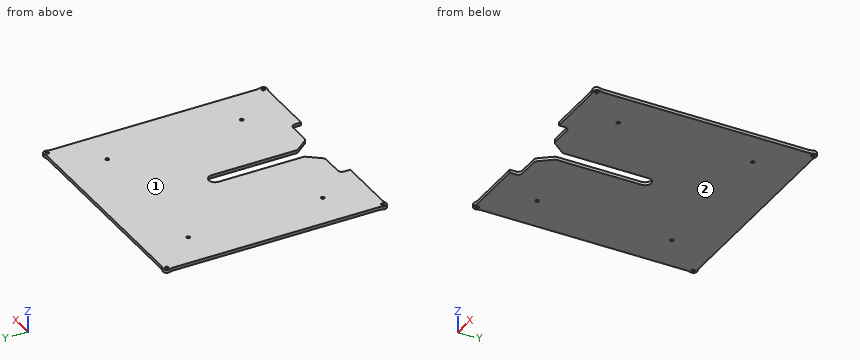
from build123d import *

# Parameters (mm, degrees)
SKETCH1_R           = 1.6
BOSS_EXTRUDE1_DEPTH = 3
CUT_EXTRUDE1_DEPTH  = 4
CUT_EXTRUDE3_DEPTH  = 4
FILLET1_R           = 4
SKETCH3_R           = 1.6
CUT_EXTRUDE2_DEPTH  = 4


with BuildPart() as part:
    # Sketch1 → Boss-Extrude1 (new body)
    with BuildSketch(Plane.XY):
        with BuildLine():
            Line((-107, 98.923010333), (-107, -98.923010333))
            ThreePointArc((-107, -98.923010333), (-107.201661971, -101.11372249), (-107.799869959, -103.230804092))
            ThreePointArc((-107.799869959, -103.230804092), (-107, -107), (-103.230804092, -107.799869959))
            ThreePointArc((-103.230804092, -107.799869959), (-101.11372249, -107.201661971), (-98.923010333, -107))
            Line((-98.923010333, -107), (-43, -107))
            Line((-43, -107), (-43, -101))
            ThreePointArc((-43, -101), (-41.828427125, -98.171572875), (-39, -97))
            Line((-39, -97), (39, -97))
            ThreePointArc((39, -97), (41.828427125, -98.171572875), (43, -101))
            Line((43, -101), (43, -107))
            Line((43, -107), (98.923010333, -107))
            ThreePointArc((98.923010333, -107), (101.11372249, -107.201661971), (103.230804092, -107.799869959))
            ThreePointArc((103.230804092, -107.799869959), (107, -107), (107.799869959, -103.230804092))
            ThreePointArc((107.799869959, -103.230804092), (107.201661971, -101.11372249), (107, -98.923010333))
            Line((107, -98.923010333), (107, 98.923010333))
            ThreePointArc((107, 98.923010333), (107.201661971, 101.11372249), (107.799869959, 103.230804092))
            ThreePointArc((107.799869959, 103.230804092), (107, 107), (103.230804092, 107.799869959))
            ThreePointArc((103.230804092, 107.799869959), (101.11372249, 107.201661971), (98.923010333, 107))
            Line((98.923010333, 107), (-98.923010333, 107))
            ThreePointArc((-98.923010333, 107), (-101.11372249, 107.201661971), (-103.230804092, 107.799869959))
            ThreePointArc((-103.230804092, 107.799869959), (-107, 107), (-107.799869959, 103.230804092))
            ThreePointArc((-107.799869959, 103.230804092), (-107.201661971, 101.11372249), (-107, 98.923010333))
        make_face()
        with Locations((-104.5, -104.5)):
            Circle(SKETCH1_R, mode=Mode.SUBTRACT)
        with Locations((-104.5, 104.5)):
            Circle(SKETCH1_R, mode=Mode.SUBTRACT)
        with Locations((104.5, 104.5)):
            Circle(SKETCH1_R, mode=Mode.SUBTRACT)
        with Locations((104.5, -104.5)):
            Circle(SKETCH1_R, mode=Mode.SUBTRACT)
    extrude(amount=BOSS_EXTRUDE1_DEPTH)

    # Sketch2 → Cut-Extrude1 (cut, through all)
    with BuildSketch(Plane(origin=(0, 0, 0), x_dir=(-1, 0, 0), z_dir=(0, 0, -1))):
        with BuildLine():
            Line((6, -97), (-6, -97))
            Line((-6, -97), (-6, 0))
            ThreePointArc((-6, 0), (0, 6), (6, 0))
            Line((6, 0), (6, -97))
        make_face()
    extrude(amount=-CUT_EXTRUDE1_DEPTH, mode=Mode.SUBTRACT)

    # Sketch4 → Cut-Extrude3 (cut, through all)
    with BuildSketch(Plane.XY.offset(3)):
        Polygon((-17, -97), (17, -97), (6, -83), (-6, -83), align=None)
    extrude(amount=-CUT_EXTRUDE3_DEPTH, mode=Mode.SUBTRACT)

    # Fillet1
    fillet1_edges = [part.edges().sort_by_distance(p)[0] for p in [
        (-17, -97, 1.5),
        (-6, -83, 1.5),
        (6, -83, 1.5),
        (17, -97, 1.5),
    ]]
    fillet(fillet1_edges, radius=FILLET1_R)

    # Sketch3 → Cut-Extrude2 (cut, through all)
    with BuildSketch(Plane.XY.offset(3)):
        with Locations((-71, 65)):
            Circle(SKETCH3_R)
        with Locations((71, 65)):
            Circle(SKETCH3_R)
        with Locations((71, -65)):
            Circle(SKETCH3_R)
        with Locations((-71, -65)):
            Circle(SKETCH3_R)
    extrude(amount=-CUT_EXTRUDE2_DEPTH, mode=Mode.SUBTRACT)


solid = part.part
Verification items for the finished model (mm, model axes). Face numbers are marked on the shaded views. Give positions to 0.01 mm unless a question says otherwise; leave off trailing zeros. Order: outer loops, then holes, each group sorted by start corner. A loop starts at its lowest first (then second) coordinate and runs counter-clockwise, first axis right, second up. Notation, with made-up numbers: M 89,-24 L 136,-24 A9 cw 136,-18 Z; hole C -14.75,73 d11. An arc over 180 degrees is marked long. Answer as a JSON object with one key per item and string values. Group by question number.
1) Cross-section at B-B (z = 0.9). Give the number of separate pieces and of enclosed holes in the cut face, then the cut area to 3 significant figures.
2) Mould release check, pull along Z, two halves, no side actions. Record for the marked faces 1 and 2: released by +Z, released by -Z, zero draft, split by the parting line, or undercut.
3) Cross-section at D-D (y = -93). Enter the section's corners in (x, z), then the cut area to 3 significant figures.
4) Cross-section at C-C (x = 35). Enter the section's corners in (y, z).
5) Scan lines: line 1 along X through (y, z) = (-104.5, 2.3); line 2 along Y through (x, z) = (71, 1.6); line 3 along X through (y, z) = (-65, 1.7). Record each from-to range of solid material in increasing order. Write a range as [from, to].
6) Depth check by flat-ended pin: pin 1 Ø3.5 at (x, y) = (-104.5, 104.5) entering from +Z; pin 2 Ø3 at (x, y) = (-71, -65) entering from +Z; pin 3 Ø0.9 at (y, z) = (-102.5, 2) entering from -X; pin 4 Ø0.9 at (x, z) = (-33.5, 1.5) entering from -Y. Enter the tip coordinate at first touch or a pass-through.
7) Cross-section at A-A (y = -27.5). Enter the section's corners in (x, z), then the cut area to 3 significant figures.
Result sheet:
{
 "1": {"separate pieces": "1", "enclosed holes": "8", "area": "43,500 mm2"},
 "2": {"face 1": "released by +Z", "face 2": "released by -Z"},
 "3": {"outline": "M -107,0 L -13.86,0 L -13.86,3 L -107,3 Z; M 13.86,0 L 107,0 L 107,3 L 13.86,3 Z", "area": "559 mm2"},
 "4": {"outline": "M -97,0 L 107,0 L 107,3 L -97,3 Z"},
 "5": {"line 1": "x = [-108.04, -106.1], [-102.9, -43], [43, 102.9], [106.1, 108.04]", "line 2": "y = [-107, -66.6], [-63.4, 63.4], [66.6, 107]", "line 3": "x = [-107, -72.6], [-69.4, -6], [6, 69.4], [72.6, 107]"},
 "6": {"pin 1": "stops at z = 3", "pin 2": "passes through", "pin 3": "stops at x = -107.7", "pin 4": "stops at y = -97"},
 "7": {"outline": "M -107,0 L -6,0 L -6,3 L -107,3 Z; M 6,0 L 107,0 L 107,3 L 6,3 Z", "area": "606 mm2"}
}
